Source: CAD feature listing. Evaluate the final solid. Frame: model axes, mm. A direction names the side the tool comes from. Give positions to 0.01 mm unless a question says otherwise; leave off trailing zeros. Write each loop counter-clockwise with the first axis right and the second up, starting at its lowest first coordinate (ties: lowest second). Pieces come first, ordered by that corner, then holes. Notation, with made-up numbers: (43, 38.25) -> (81, 38.25) arc R22 cw to (81, 69.25) -> close; hole circle Ø10 at (1.25, 15.25). An arc over 180 degrees is marked (long way). Write item = value, one per line.
from build123d import *

# Parameters (mm, degrees)
F2_DEPTH  = 15
F3_R      = 2
F4_R      = 1
F7_DEPTH  = 15
F8_W      = 3.7031254775
F8_H      = 13
F9_DEPTH  = 25
F10_R     = 1.25
F11_DEPTH = 13


with BuildPart() as f2:
    # F1 (on Front) → F2 (new body)
    with BuildSketch(Plane.XZ):
        Polygon((10, 22.2655313462), (0, 12.2655313462), (0, -9.6663414017), (7.7085571088, -9.6663414017), (28.4380931407, 0), (30, 1.5619068593), (30, 30.3336585983), (10, 30.3336585983), align=None)
    extrude(amount=F2_DEPTH)

    # F3
    f3_edges = [f2.edges().sort_by_distance(p)[0] for p in [
        (0, -7.5, 12.265531),
        (0, -7.5, -9.666341),
    ]]
    fillet(f3_edges, radius=F3_R)

    # F4
    f4_edges = [f2.edges().sort_by_distance(p)[0] for p in [
        (5.292893, -15, 17.558425),
        (10, -15, 26.299595),
        (10, 0, 26.299595),
        (5.292893, 0, 17.558425),
        (18.073325, -15, -4.833171),
        (30, -15, 15.947783),
        (29.219047, -15, 0.780953),
        (29.219047, 0, 0.780953),
        (30, 0, 15.947783),
        (18.073325, 0, -4.833171),
        (0.152241, 0, 12.202471),
        (0, 0, 1.885381),
        (0.585786, 0, -9.080555),
        (4.854279, 0, -9.666341),
        (0.152241, -15, 12.202471),
        (0, -15, 1.885381),
        (0.585786, -15, -9.080555),
        (4.854279, -15, -9.666341),
    ]]
    fillet(f4_edges, radius=F4_R)

    # F6 (on Front) → F7 (join)
    with BuildSketch(Plane.XZ):
        with BuildLine():
            Line((18.75, 30.3336585983), (21.25, 30.3336585983))
            Line((21.25, 30.3336585983), (21.25, 36.8336585983))
            ThreePointArc((21.25, 36.8336585983), (20, 38.0836585983), (18.75, 36.8336585983))
            Line((18.75, 36.8336585983), (18.75, 30.3336585983))
        make_face()
    extrude(amount=F7_DEPTH)

    # F8 (on face) → F9 (cut)
    with BuildSketch(Plane.XY.offset(30.3336585983)):
        with Locations((20.149352029, -7.5)):
            Rectangle(F8_W, F8_H)
    extrude(amount=F9_DEPTH, mode=Mode.SUBTRACT)

    # F10 (on face) → F11 (join)
    with BuildSketch(Plane.XZ.offset(1)):
        with Locations((20, 36.8336585983)):
            Circle(F10_R)
    extrude(amount=F11_DEPTH)


solid = f2.part
(1) Access query for faces 1 (the face through (10.301, -0.285, 26.033)), 2 (the face through (21.25, -0.5, 33.5)), 3 (the face through (10.285, -14.699, 26.033)). Directions: +Z, -Z, +X, -X, +Y, -Y. A direction counts if a zero-diameter tool reaches every point of the face in a straight line with its end or side. Return the directions, or none.
Values follow:
face_1 = +Z, -X, +Y
face_2 = +Z, +X, +Y, -Y
face_3 = +Z, -X, -Y
(2) Section query A-A (y = -4.75). Return loops of the section in (x, z).
Values follow:
outline = (0, -7.67) arc R2 ccw to (2, -9.67) -> (7.71, -9.67) -> (28.44, 0) -> (30, 1.56) -> (30, 30.33) -> (10, 30.33) -> (10, 22.27) -> (0.59, 12.85) arc R2 ccw to (0, 11.44) -> close; circle Ø2.5 at (20, 36.83)
(3) Pull-direction query (Z, two-part tool) for faces 4 (the face through (5.359, -7.409, 17.624)), 5 (the face through (10, -7, 26)), 6 (the face through (19.837, -7.395, 38.073)), 7 (the face through (4.89, -14.7, -9.38)); classes: pulls with the +Z half, pulls with the -Z half, needs draft (parallel to the pull), parting line crosses it, or undercut.
Values follow:
face_4 = pulls with the +Z half
face_5 = needs draft
face_6 = undercut
face_7 = pulls with the -Z half
(4) Section query B-B (z = 26.5). Return loops of the section in (x, y).
Values follow:
outline = (10, -14) arc R1 ccw to (11, -15) -> (29, -15) arc R1 ccw to (30, -14) -> (30, -1) arc R1 ccw to (29, 0) -> (11, 0) arc R1 ccw to (10, -1) -> close
(5) Material intervals for line 1 (X direction, y = -12.5, z = 24); line 2 (X direction, y = -6, z = 20); line 3 (Z direction, x = 8.5, y = -14.25), sorted ascending.
Values follow:
line_1 = 10 to 30
line_2 = 7.73 to 30
line_3 = -9.26 to 20.72
(6) First-contact query: pin 1 (4 mm diameter, centred on y = -10.5, z = 25, fed in from -X); pin 2 (0.5 mm diameter, centred on y = -14.5, z = 32.5, fed in from +X); pin 3 (0.8 mm diameter, centred on y = -14.5, z = 33.5, fed in from -X); pin 4 (1.2 mm diameter, centred on x = 20.5, z = 33, fed in from +Y). Flat tips, straight axial feed; report the tip coordinate or a pass-through.
Values follow:
pin_1 = 10
pin_2 = 21.25
pin_3 = 18.75
pin_4 = 0
